Geometry check sheet. Reference: the model listing, model coordinates, mm. Face numbers are marked on the shaded views. A direction names the side the tool comes from. Give positions to 0.01 mm unless a question says otherwise; leave off trailing zeros. Loops run counter-clockwise (first coordinate to the right, second up) from the corner with the lowest first, then second, coordinate; pieces in that order, holes last.
1. Cross-section at C-C, the plane y = -91. Record the cut outline in (x, z), plus the area to 3 significant figures.
2. Cross-section at B-B, the plane z = 24. Record the cut outline in (x, y).
3. Material ranges on L1, parallel to Y at x = 64.5, z = 23.5; L2, parallel to X at y = -195, z = 23; L3, parallel to X at y = -131, z = 1.55, recorded low to high.
4. Cross-section at A-A, the plane x = 44. Record the cut outline in (y, z), plus the area to 3 significant figures.
5. Tool access check on the marked faces 1, 2 and 3. Record the directions out of +Z, -Z, +X, -X, +Y, -Y that give a thin tool (end or side, any length) a straight path to the whole face; none if there is none.
6. Release check for a two-part mould opening along X. For the marked faces 4, 5 and 6 record: +X half, -X half, draft (parallel to the pull), parting line (faces both ways), or undercut.
7. Cross-section at D-D, the plane y = -62.5. Record the cut outline in (x, z).
8. Go/stop test with flat-tipped pins: pin 1 Ø9.5 at (x, y) = (18, -91) entering from -Z; pin 2 Ø12 at (x, z) = (170, 22) entering from -Y; pin 3 Ø8 at (x, z) = (28.5, 5.5) entering from +Y; pin 4 Ø1 at (x, y) = (116, -153.5) entering from +Z. Record where each tip stops, or that it passes through.
from build123d import *

# Parameters (mm, degrees)
F1_DEPTH  = 222
F2_SIZE   = 10
F3_SIZE   = 10
F4_SIZE   = 8
F6_W      = 202
F6_H      = 35
F7_DEPTH  = 55
F8_SIZE   = 10
F9_SIZE   = 10
F10_SIZE  = 5
F11_SIZE  = 8
F12_T     = -2.5
F5_R      = 3
F13_DEPTH = 35.001


with BuildPart() as f1:
    # F0 (on Front) → F1 (new body)
    with BuildSketch(Plane.XZ):
        Polygon((0, 0), (10, 0), (140, 0), (150, 0), (150, 10), (150, 35), (0, 35), (0, 10), align=None)
    extrude(amount=F1_DEPTH)

    # F2
    f2_edges = [f1.edges().sort_by_distance(p)[0] for p in [
        (0, -222, 17.5),
        (150, -222, 17.5),
        (150, 0, 17.5),
        (0, 0, 17.5),
    ]]
    chamfer(f2_edges, length=F2_SIZE)

    # F3 (call 1 of 3: OpenCascade refuses the feature's edges together)
    f3_edges = [f1.edges().sort_by_distance(p)[0] for p in [
        (75, -222, 0),
    ]]
    chamfer(f3_edges, length=F3_SIZE)

    # F3#2 (call 2 of 3)
    f3_2_edges = [f1.edges().sort_by_distance(p)[0] for p in [
        (75, 0, 0),
    ]]
    chamfer(f3_2_edges, length=F3_SIZE)

    # F3#3 (call 3 of 3)
    f3_3_edges = [f1.edges().sort_by_distance(p)[0] for p in [
        (0, -111, 0),
    ]]
    chamfer(f3_3_edges, length=F3_SIZE)

    # F4
    f4_edges = [f1.edges().sort_by_distance(p)[0] for p in [
        (7.5, -214.5, 2.5),
        (7.5, -7.5, 2.5),
    ]]
    chamfer(f4_edges, length=F4_SIZE)

    # F6 (on face) → F7 (join)
    with BuildSketch(Plane.YZ.offset(150)):
        with Locations((-111, 17.5)):
            Rectangle(F6_W, F6_H)
    extrude(amount=F7_DEPTH)

    # F8
    f8_edges = [f1.edges().sort_by_distance(p)[0] for p in [
        (205, -111, 0),
        (177.5, -212, 0),
        (177.5, -10, 0),
    ]]
    chamfer(f8_edges, length=F8_SIZE)

    # F9
    f9_edges = [f1.edges().sort_by_distance(p)[0] for p in [
        (205, -212, 22.5),
        (205, -10, 22.5),
    ]]
    chamfer(f9_edges, length=F9_SIZE)

    # F10
    f10_edges = [f1.edges().sort_by_distance(p)[0] for p in [
        (145, -217, 5),
        (145, -5, 5),
    ]]
    chamfer(f10_edges, length=F10_SIZE)

    # F11
    f11_edges = [f1.edges().sort_by_distance(p)[0] for p in [
        (197.5, -17.5, 2.5),
        (197.5, -204.5, 2.5),
    ]]
    chamfer(f11_edges, length=F11_SIZE)

    # F12
    f12_openings = [f1.faces().sort_by_distance(p)[0] for p in [
        (100.529547, -111, 35),
    ]]
    offset(amount=F12_T, openings=f12_openings, kind=Kind.INTERSECTION)

    # F5 (on face) → F13 (cut, through all)
    with BuildSketch(Plane(origin=(0, 0, 0), x_dir=(1, 0, 0), z_dir=(0, 0, -1))):
        with Locations((18, 131)):
            Circle(F5_R)
        with Locations((44, 131)):
            Circle(F5_R)
        with Locations((44, 91)):
            Circle(F5_R)
        with Locations((18, 91)):
            Circle(F5_R)
    extrude(amount=-F13_DEPTH, mode=Mode.SUBTRACT)


solid = f1.part
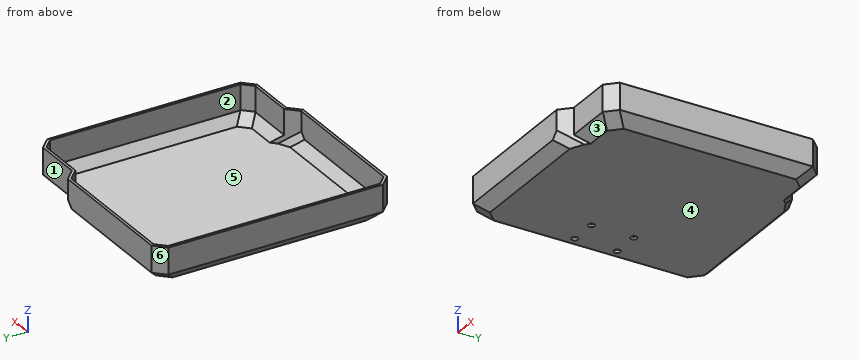
Result:
1. outline: (0, 10) - (10, 0) - (15, 0) - (15, 2.5) - (11.04, 2.5) - (2.5, 11.04) - (2.5, 35) - (0, 35) - close; (21, 0) - (41, 0) - (41, 2.5) - (21, 2.5) - close; (47, 0) - (195, 0) - (205, 10) - (205, 35) - (202.5, 35) - (202.5, 11.04) - (193.96, 2.5) - (47, 2.5) - close
1. area: 618 mm2
2. outline: (0, -212) - (10, -222) - (140, -222) - (150, -212) - (195, -212) - (205, -202) - (205, -20) - (195, -10) - (150, -10) - (140, 0) - (10, 0) - (0, -10) - close; hole (2.5, -210.96) - (11.04, -219.5) - (138.96, -219.5) - (148.96, -209.5) - (193.96, -209.5) - (202.5, -200.96) - (202.5, -21.04) - (193.96, -12.5) - (148.96, -12.5) - (138.96, -2.5) - (11.04, -2.5) - (2.5, -11.04) - close
3. L1: y = -222 to -219.5, -2.5 to 0
3. L2: x = 0 to 2.5, 202.5 to 205
3. L3: x = 8.45 to 15, 21 to 41, 47 to 196.55
4. outline: (-222, 10) - (-212, 0) - (-134, 0) - (-134, 2.5) - (-210.96, 2.5) - (-219.5, 11.04) - (-219.5, 35) - (-222, 35) - close; (-128, 0) - (-94, 0) - (-94, 2.5) - (-128, 2.5) - close; (-88, 0) - (-10, 0) - (0, 10) - (0, 35) - (-2.5, 35) - (-2.5, 11.04) - (-11.04, 2.5) - (-88, 2.5) - close
4. area: 660 mm2
5. face 1: +Z, -Z, +X, +Y
5. face 2: +Z
5. face 3: -Z, +X, -Y
6. face 4: draft
6. face 5: undercut
6. face 6: -X half
7. outline: (0, 10) - (10, 0) - (195, 0) - (205, 10) - (205, 35) - (202.5, 35) - (202.5, 11.04) - (193.96, 2.5) - (11.04, 2.5) - (2.5, 11.04) - (2.5, 35) - (0, 35) - close
8. pin 1: stops at z = 0
8. pin 2: stops at y = -212
8. pin 3: stops at y = -0.5
8. pin 4: stops at z = 2.5
